Geometry: final body of the model. Coordinates: model frame, mm. A direction names the side the tool comes from. Coordinates: 2 decimals unless noted, no trailing zeros. Loops run counter-clockwise (first coordinate to the right, second up) from the corner with the lowest first, then second, coordinate; pieces in that order, holes last. Notation, with made-up numbers: (18.5, 81) -> (34.5, 81) arc R16 cw to (34.5, 90) -> close; hole circle Ø1 at (45.25, 73). An arc over 180 degrees is marked (long way). One line per item, written item: value. Start each with the question number.
Autodesk Fusion 360 part; units mm, degrees
sketch "Sketch1" plane through (0, 0, 0) normal (0, 0, 1) x (1, 0, 0) in component "Main plate"
  line L0 (12, -33.0003) -> (12, -49)
  line L1 (-14.5, -33.0003) -> (14.5, -33.0003)
  line L2 (14.5, 33) -> (-14.5, 33)
  line L3 (-9, 52) -> (9, 52)
  line L4 (-12, 33) -> (-12, 49)
  line L5 (16.5, -31.0003) -> (16.5, 31)
  line L6 (-12, -49) -> (-12, -33.0003)
  circle A0 centre (0, -48.5) radius 1.39
  circle A1 centre (0, 48.5) radius 1.39
  line L7 (9, -52) -> (-9, -52)
  line L8 (12, 49) -> (12, 33)
  arc A2 (-14.5, 33) -> (-16.5, 31) centre (-14.5, 31) ccw
  line L9 (-16.5, 31) -> (-16.5, -31.0003)
  arc A3 (16.5, 31) -> (14.5, 33) centre (14.5, 31) ccw
  arc A4 (14.5, -33.0003) -> (16.5, -31.0003) centre (14.5, -31.0003) ccw
  arc A5 (-16.5, -31.0003) -> (-14.5, -33.0003) centre (-14.5, -31.0003) ccw
  arc A6 (-12, -49) -> (-9, -52) centre (-9, -49) ccw
  arc A7 (9, -52) -> (12, -49) centre (9, -49) ccw
  arc A8 (-9, 52) -> (-12, 49) centre (-9, 49) ccw
  arc A9 (12, 49) -> (9, 52) centre (9, 49) ccw
  line L10 (-14.5, -35.8766) -> (14.5, -35.8766)
  arc A10 (14.5, -35.8766) -> (19.3763, -31.0003) centre (14.5, -31.0003) ccw
  line L11 (19.3763, -31.0003) -> (19.3763, 31)
  arc A11 (19.3763, 31) -> (14.5, 35.8763) centre (14.5, 31) ccw
  line L12 (14.5, 35.8763) -> (-14.5, 35.8763)
  arc A12 (-14.5, 35.8763) -> (-19.3763, 31) centre (-14.5, 31) ccw
  line L13 (-19.3763, 31) -> (-19.3763, -31.0003)
  arc A13 (-19.3763, -31.0003) -> (-14.5, -35.8766) centre (-14.5, -31.0003) ccw
  line L14 (-4, 39.75) -> (4, 39.75)
  arc A14 (4, 39.75) -> (4, 44.25) centre (4, 42) ccw
  line L15 (4, 44.25) -> (-4, 44.25)
  arc A15 (-4, 44.25) -> (-4, 39.75) centre (-4, 42) ccw
  line L16 (-4, 42) -> (4, 42) construction
  line L17 (-4, -42) -> (4, -42) construction
  arc A16 (4, -44.25) -> (4, -39.75) centre (4, -42) ccw
  line L18 (-4, -44.25) -> (4, -44.25)
  arc A17 (-4, -39.75) -> (-4, -44.25) centre (-4, -42) ccw
  line L19 (4, -39.75) -> (-4, -39.75)
  line L20 (-14.5, -31.5003) -> (14.5, -31.5003)
  arc A18 (14.5, -31.5003) -> (15, -31.0003) centre (14.5, -31.0003) ccw
  line L21 (15, -31.0003) -> (15, 31)
  arc A19 (15, 31) -> (14.5, 31.5) centre (14.5, 31) ccw
  line L22 (14.5, 31.5) -> (-14.5, 31.5)
  arc A20 (-14.5, 31.5) -> (-15, 31) centre (-14.5, 31) ccw
  line L23 (-15, 31) -> (-15, -31.0003)
  arc A21 (-15, -31.0003) -> (-14.5, -31.5003) centre (-14.5, -31.0003) ccw
  line L24 (9, -0.75) -> (-9, -0.75)
  line L25 (-9, -0.75) -> (-9, 0.75)
  line L26 (-9, 0.75) -> (9, 0.75)
  line L27 (9, 0.75) -> (9, -0.75)
  line L28 (9, 3.75) -> (9, 2.25)
  line L29 (9, 2.25) -> (-9, 2.25)
  line L30 (-9, 2.25) -> (-9, 3.75)
  line L31 (-9, 3.75) -> (9, 3.75)
  line L32 (-9, 5.25) -> (-9, 6.75)
  line L33 (-9, 6.75) -> (9, 6.75)
  line L34 (9, 5.25) -> (-9, 5.25)
  line L35 (9, 6.75) -> (9, 5.25)
  line L36 (-9, -2.25) -> (9, -2.25)
  line L37 (9, -2.25) -> (9, -3.75)
  line L38 (-9, -3.75) -> (-9, -2.25)
  line L39 (9, -3.75) -> (-9, -3.75)
  line L40 (9, -5.25) -> (9, -6.75)
  line L41 (-9, -5.25) -> (9, -5.25)
  line L42 (-9, -6.75) -> (-9, -5.25)
  line L43 (9, -6.75) -> (-9, -6.75)
  line L44 (12, -9.5) -> (-12, -9.5)
  line L45 (-12, -9.5) -> (-12, 9.5)
  line L46 (-12, 9.5) -> (12, 9.5)
  line L47 (12, 9.5) -> (12, -9.5)
  line L48 (13, -10.5) -> (-13, -10.5)
  line L49 (-13, -10.5) -> (-13, 10.5)
  line L50 (-13, 10.5) -> (13, 10.5)
  line L51 (13, 10.5) -> (13, -10.5)
  circle A22 centre (10, 13.5) radius 1.45
  circle A23 centre (10, -20) radius 1.45
  circle A24 centre (10, 13.5) radius 2.95
  circle A25 centre (10, -20) radius 2.95
  point P0 (10, 0)
  point P1 (10, 0)
  point P2 (0, 42)
  point P3 (0, -42)
  point P4 (0, 3)
  point P5 (0, 3)
  point P6 (0, 3)
  point P7 (0, 3)
  point P8 (0, 6)
  point P9 (0, 6)
  point P10 (0, 6)
  point P11 (0, 6)
  point P12 (0, -3)
  point P13 (0, -3)
  point P14 (0, -3)
  point P15 (0, -3)
  point P16 (0, -6)
  point P17 (0, -6)
  point P18 (0, -6)
  point P19 (0, -6)
  point P20 (10, 0)
  dimension "d15" = 2
  dimension "d16" = 2
  dimension "d17" = 3
  dimension "d18" = 3
  dimension "d19" = 3
  dimension "d20" = 3
  dimension "d26" = 4.5
  dimension "d27" = 4.5
  dimension "d54" = 2.9
  dimension "d55" = 2.9
  dimension "d56" = 1.5
  dimension "d57" = 1.5
  dimension "d66" = 2.78
  dimension "d67" = 2.78
extrude "Extrude1" add sketch "Sketch1" along normal blind 5 contours L1 L2 L5 A2 L9 A3 A4 A5 | L20 A18 L21 A19 L22 A20 L23 A21 | L24 L25 L26 L27 | L28 L29 L30 L31 | L32 L33 L34 L35 | L36 L37 L38 L39 | L40 L41 L42 L43 | L44 L45 L46 L47 | L48 L49 L50 L51 | A22 | A23 | A24 | A25 makes body 1 in component "Main plate"
extrude "Extrude2" add sketch "Sketch1" against normal blind 1.5 separate body contours L0 L1 L2 L5 L8 A3 A4 L10 A10 L11 A11 L12 | L0 L1 L6 L10 | L0 L6 L7 A6 A7 L10 | L1 L2 L4 L6 A2 L9 A5 L10 L12 A12 L13 A13 | L2 L4 L8 L12 | L3 L4 L8 A8 A9 L12 makes body 2 in component "Main plate"
extrude "Extrude3" cut sketch "Sketch1" against normal through all contours L14 A14 L15 A15 bodies 2 in component "Main plate"
extrude "Extrude4" cut sketch "Sketch1" against normal through all contours A16 L18 A17 L19 bodies 2 in component "Main plate"
extrude "Extrude5" add sketch "Sketch1" against normal blind 1.5 contours L1 L2 L5 A2 L9 A3 A4 A5 | L20 A18 L21 A19 L22 A20 L23 A21 | L24 L25 L26 L27 | L28 L29 L30 L31 | L32 L33 L34 L35 | L36 L37 L38 L39 | L40 L41 L42 L43 | L44 L45 L46 L47 | L48 L49 L50 L51 | A22 | A23 | A24 | A25 bodies 1 2 in component "Main plate"
extrude "Extrude6" cut sketch "Sketch1" along normal blind 3.5 contours L20 A18 L21 A19 L22 A20 L23 A21 | L24 L25 L26 L27 | L28 L29 L30 L31 | L32 L33 L34 L35 | L36 L37 L38 L39 | L40 L41 L42 L43 | L44 L45 L46 L47 | L48 L49 L50 L51 | A22 | A23 | A24 | A25 bodies 1 in component "Main plate"
extrude "Extrude7" add sketch "Sketch1" along normal blind 3.5 separate body contours L20 A18 L21 A19 L22 A20 L23 A21 | L24 L25 L26 L27 | L28 L29 L30 L31 | L32 L33 L34 L35 | L36 L37 L38 L39 | L40 L41 L42 L43 | L44 L45 L46 L47 | L48 L49 L50 L51 | A22 | A23 | A24 | A25 makes body 3 in component "Main plate"
extrude "Extrude8" add sketch "Sketch1" against normal blind 1.5 contours L20 A18 L21 A19 L22 A20 L23 A21 | L24 L25 L26 L27 | L28 L29 L30 L31 | L32 L33 L34 L35 | L36 L37 L38 L39 | L40 L41 L42 L43 | L44 L45 L46 L47 | L48 L49 L50 L51 | A22 | A23 | A24 | A25 bodies 3 in component "Main plate"
combine "Combine1" operation cut target body 1 tool bodies 3 in component "Main plate"
extrude "Extrude9" add sketch "Sketch1" along normal blind 13 separate body contours L24 L25 L26 L27 | L28 L29 L30 L31 | L32 L33 L34 L35 | L36 L37 L38 L39 | L40 L41 L42 L43 makes body 4 at (3, -0.75, 4.3333) makes body 5 at (-3, -2.25, 4.3333) makes body 6 at (3, 2.25, 4.3333) makes body 7 at (3, -6.75, 4.3333) makes body 8 at (-3, 6.75, 4.3333) in component "Main plate"
combine "Combine2" operation cut target body 1 tool bodies 8 6 4 5 7 in component "Main plate"
extrude "Extrude10" add sketch "Sketch1" along normal blind 4 contours L48 L49 L50 L51 bodies 1 in component "Main plate"
extrude "Extrude11" add 1 faces at (-4, -10.1667, 0) along direction (0, 0, -1) blind 4.5 on bodies 1 bodies 1 in component "Main plate"
extrude "Extrude12" add sketch "Sketch1" along normal blind 3.5 separate body contours A24 makes body 9 in component "Main plate"
extrude "Extrude13" add sketch "Sketch1" against normal blind 6.5 contours A24 bodies 9 in component "Main plate"
extrude "Extrude14" add sketch "Sketch1" along normal blind 3.5 separate body contours A25 makes body 10 in component "Main plate"
extrude "Extrude15" add sketch "Sketch1" against normal blind 6.5 contours A25 bodies 10 in component "Main plate"
combine "Combine3" operation add target body 1 tool bodies 9 10 in component "Main plate"
move_face "OffsetFaces1" offset 1.5 1 faces at (12.439, 13.3534, -6.5) on bodies 1 in component "Main plate"
move_face "OffsetFaces2" offset 1.5 1 faces at (12.4336, -20.2186, -6.5) on bodies 1 in component "Main plate"
component "Main plate" placed x (1, 0, 0) y (0, 1, 0) z (0, 0, 1) at (0, 0, 0)
1. Draft query along X for faces 1 (the face through (-6.25, -41.95, -0.74)), 2 (the face through (0, 9.5, 0)), 3 (the face through (0, 8, 5)), 4 (the face through (-17.986, -34.41, -0.74)). Return one class per face: released by +X, released by -X, zero draft, split by the parting line, or undercut.
2. Section A-A on z = -3. Return the cut outline in (x, y).
3. Pin query (flat end, axial travel): pin 1 Ø2 at (y, z) = (-5, 1.5) entering from -X; pin 2 Ø1.2 at (x, z) = (1, 4) entering from -Y; pin 3 Ø4 at (y, z) = (-4.5, 2.5) entering from +X. Return the tip coordinate at first contact, or that it passes through.
4. Section B-B on y = -42. Return the cut outline in (x, z), plus the area to 4 significant figures.
5. Set-up query: faces 5 (the face through (-6.25, 42.05, -0.74)), 6 (the face through (8.55, 13.44, -2.33)), 7 (the face through (-17, 1, 0)), 8 (the face through (0, 33, 2)), 9 (the face through (11.3, -21.3, -8)). Return all of +Z, -Z, +X, -X, +Y, -Y with unobstructed straight access to the full face (end or side cutting, diameter ignored); none if empty.
6. Section D-D on x = 0. Count the separate pieces of the cut face and the enclosed holes in it, plus the area to 3 significant figures.
7. Section C-C on y = 13.5. Return the cut outline in (x, z), plus the area to 3 significant figures.
8. Line query: L1, parallel to Y at x = 0, z = 2.25; L2, parallel to X at y = -9, z = -3.5; L3, parallel to Y at x = 11.5, z = -1.75. Output: solid intervals per line, ascending. Write a range as [from, to].
Checks:
1. face 1: undercut
1. face 2: undercut
1. face 3: zero draft
1. face 4: released by -X
2. outline: (-13, -10.5) -> (13, -10.5) -> (13, 10.5) -> (-13, 10.5) -> close; circle Ø5.9 at (10, -20); circle Ø5.9 at (10, 13.5); hole (-12, -9.5) -> (12, -9.5) -> (12, 9.5) -> (-12, 9.5) -> close; hole circle Ø2.9 at (10, -20); hole circle Ø2.9 at (10, 13.5)
3. pin 1: x = -16.5
3. pin 2: y = -33
3. pin 3: x = 16.5
4. outline: (-12, -1.5) -> (-6.25, -1.5) -> (-6.25, 0) -> (-12, 0) -> close; (6.25, -1.5) -> (12, -1.5) -> (12, 0) -> (6.25, 0) -> close
4. area: 17.25 mm²
5. face 5: +Z, -Z
5. face 6: -Z
5. face 7: +Z
5. face 8: +Z, +X, -X, +Y
5. face 9: -Z, +X, -X, +Y, -Y
6. separate pieces: 10
6. enclosed holes: 0
6. area: 154 mm²
7. outline: (-19.38, -1.5) -> (-15, -1.5) -> (-15, 3.5) -> (7.05, 3.5) -> (7.05, -8) -> (8.55, -8) -> (8.55, 3.5) -> (11.45, 3.5) -> (11.45, -8) -> (12.95, -8) -> (12.95, 3.5) -> (15, 3.5) -> (15, -1.5) -> (19.38, -1.5) -> (19.38, 0) -> (16.5, 0) -> (16.5, 5) -> (-16.5, 5) -> (-16.5, 0) -> (-19.38, 0) -> close
7. area: 108 mm²
8. L1: [-33, -31.5], [-10.5, -9.5], [9.5, 10.5], [31.5, 33]
8. L2: [-13, -12], [12, 13]
8. L3: [-22.54, -17.46], [-10.5, -9.5], [9.5, 10.5], [10.96, 16.04]
